Here's the drawing with two shaded views (mm, measured from the low corner). I have some questions. Give positions to 0.01 mm unless a question says otherwise; leave off trailing zeros. Loops run counter-clockwise (first coordinate to the right, second up) from the corner with the lowest first, then second, coordinate; pieces in that order, holes last. Notation, with made-up numbers: M 82,68.25 L 137,68.25 A14 ccw 137,82.25 Z; hole C 79.25,4 d6. An arc over 180 degrees is marked long. Write item = value, one per line. Start each with the question number.
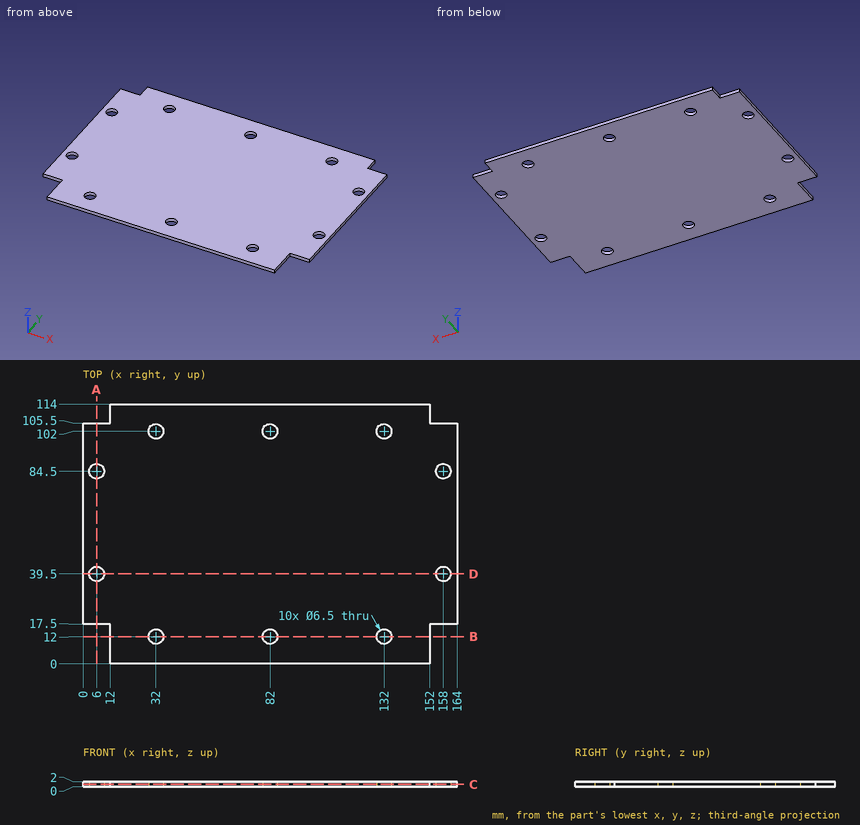
Q1. If we section it at A-A, the plane x = 6: List the corners of the cut face in (y, z) for me.
Q2. If I drill on line 1 along Y through (x, z) = (32, 0.8); line 2 along Y through (x, z) = (158, 0.55); line 3 along X through (y, z) = (11.5, 0.9), over which ranges is the centre line in solid material (lowest first)?
Q3. If we section it at D-D, the plane y = 39.5: List the corners of the cut face in (x, z) for me.
Q4. If we section it at C-C, the plane z = 0.9: State how many separate pieces and enclosed holes the cut face has, then the cut area to 3 significant figures.
Q5. If we section it at B-B, the plane y = 12: List the corners of the cut face in (x, z) for me, then the cut area to 3 significant figures.
Q6. Will these pins go through, and if not, where does the flat tip stop? pin 1 (0.6 mm diameter, centred on y = 108, z = 1, fed in from -X); pin 2 (6 mm diameter, centred on x = 158, y = 84.5, fed in from +Z); pin 3 (1 mm diameter, centred on x = 158, z = 1.5, fed in from -Y); pin 4 (1 mm diameter, centred on y = 11, z = 1, fed in from +X).
Resolved:
q1.outline = M 17.5,0 L 36.25,0 L 36.25,2 L 17.5,2 Z; M 42.75,0 L 81.25,0 L 81.25,2 L 42.75,2 Z; M 87.75,0 L 105.5,0 L 105.5,2 L 87.75,2 Z
q2.line_1 = 0 to 8.75, 15.25 to 98.75, 105.25 to 114
q2.line_2 = 17.5 to 36.25, 42.75 to 81.25, 87.75 to 105.5
q2.line_3 = 12 to 28.79, 35.21 to 78.79, 85.21 to 128.79, 135.21 to 152
q3.outline = M 0,0 L 2.75,0 L 2.75,2 L 0,2 Z; M 9.25,0 L 154.75,0 L 154.75,2 L 9.25,2 Z; M 161.25,0 L 164,0 L 164,2 L 161.25,2 Z
q4.separate_pieces = 1
q4.enclosed_holes = 10
q4.area = 17,700 mm²
q5.outline = M 12,0 L 28.75,0 L 28.75,2 L 12,2 Z; M 35.25,0 L 78.75,0 L 78.75,2 L 35.25,2 Z; M 85.25,0 L 128.75,0 L 128.75,2 L 85.25,2 Z; M 135.25,0 L 152,0 L 152,2 L 135.25,2 Z
q5.area = 241 mm²
q6.pin_1 = 12
q6.pin_2 = through
q6.pin_3 = 17.5
q6.pin_4 = 152
